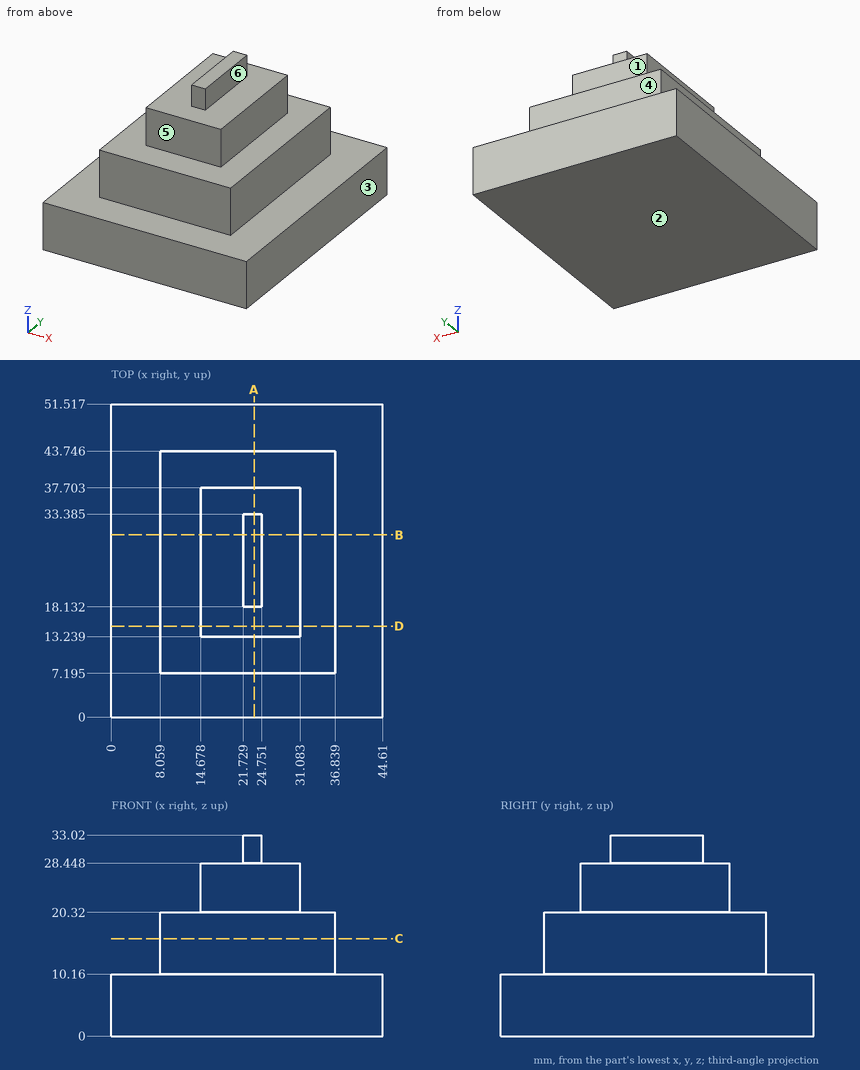
The drawing under review shows one solid part. Ordinate dimensions are in mm from its lowest x, y, z. A direction names the side the tool comes from. Coordinates: 2 decimals unless noted, no trailing zeros. Write each loop counter-clockwise with the first axis right and the second up, starting at its lowest first coordinate (ties: lowest second). Pieces come first, ordered by that corner, then holes.
1) Add section C-C (z = 16). Write out the cut boundary in (x, y) (1 decimal).
2) To check wall thickness, follow L1, parallel to X at y = 26, z = 20; L2, parallel to Z at x = 8, y = 31; L3, parallel to Z at x = 10.5, y = 32.5. State the ranges of each line that lie inside material, in increasing order.
3) Add section A-A (x = 23.5). Write out the cut boundary in (y, z) (1 decimal), plus the area to 3 significant figures.
4) Insertion check: pin 1 (9 mm diameter, centred on x = 26.5, z = 23.5, fed in from +Y); pin 2 (0.9 mm diameter, centred on x = 23.5, z = 31.5, fed in from +Y) (1 decimal); pin 3 (1.4 mm diameter, centred on y = 25.5, z = 31, fed in from +X). Each pin has a flat end and moves straight along its axis. Give the tip position at first contact, or say it passes through.
5) Machinability: for the marked faces 3, 4, 5 and 6, which of the approach directions +Z, -Z, +X, -X, +Y, -Y give a long, thin tool a straight path to every point of the face, cutting with its end or side? Answer none if there is none.
6) Add section D-D (y = 15). Write out the cut boundary in (x, z), plus the area to 3 significant figures.
7) Add section B-B (y = 30). Write out the cut boundary in (x, z).
8) Mouldability with a two-part tool opening along Z and no side actions: class the marked faces 1 and 2 as +Z half, -Z half, draft (parallel to the pull), parting line (faces both ways), or undercut.
Check result:
1. outline: (8.1, 7.2) - (36.8, 7.2) - (36.8, 43.7) - (8.1, 43.7) - close
2. L1: x = 8.06 to 36.84
2. L2: z = 0 to 10.16
2. L3: z = 0 to 20.32
3. outline: (0, 0) - (51.5, 0) - (51.5, 10.2) - (43.7, 10.2) - (43.7, 20.3) - (37.7, 20.3) - (37.7, 28.4) - (33.4, 28.4) - (33.4, 33) - (18.1, 33) - (18.1, 28.4) - (13.2, 28.4) - (13.2, 20.3) - (7.2, 20.3) - (7.2, 10.2) - (0, 10.2) - close
3. area: 1,160 mm2
4. pin 1: stops at y = 43.75
4. pin 2: stops at y = 33.4
4. pin 3: stops at x = 24.75
5. face 3: +Z, -Z, +X, +Y, -Y
5. face 4: +Z, +X, -X, +Y
5. face 5: +Z, +X, -X, -Y
5. face 6: +Z, +X, +Y, -Y
6. outline: (0, 0) - (44.61, 0) - (44.61, 10.16) - (36.84, 10.16) - (36.84, 20.32) - (31.08, 20.32) - (31.08, 28.45) - (14.68, 28.45) - (14.68, 20.32) - (8.06, 20.32) - (8.06, 10.16) - (0, 10.16) - close
6. area: 879 mm2
7. outline: (0, 0) - (44.61, 0) - (44.61, 10.16) - (36.84, 10.16) - (36.84, 20.32) - (31.08, 20.32) - (31.08, 28.45) - (24.75, 28.45) - (24.75, 33.02) - (21.73, 33.02) - (21.73, 28.45) - (14.68, 28.45) - (14.68, 20.32) - (8.06, 20.32) - (8.06, 10.16) - (0, 10.16) - close
8. face 1: draft
8. face 2: -Z half
